Work out the finished part from the listing and answer in its coordinate system (mm). Face numbers are marked on the shaded views. A direction names the side the tool comes from. Give positions to 0.01 mm unless a question says otherwise; leave off trailing zeros. Order: outer loops, then holes, each group sorted by start corner. A loop starts at its lowest first (then second) coordinate and runs counter-clockwise, first axis right, second up. Notation, with made-up numbers: M -2,-20 L 21,-20 A17 cw 21,-3 Z; hole C 25.5,-30 d9. An arc over 180 degrees is marked long. One line per item, written item: value.
Autodesk Inventor part; units mm, degrees
ref_plane "Work Plane1" through (0, -50, 20) normal (0, -1, 0) x (0, 0, -1)
ref_plane "YZ Plane" through (0, 0, 0) normal (1, 0, 0) x (0, 1, 0)
ref_plane "XZ Plane" through (0, 0, 0) normal (0, 1, 0) x (-1, 0, 0)
sketch "Sketch1" plane through (0, 0, 0) normal (1, 0, 0) x (0, 1, 0)
  arc A0 (-15, -20) -> (-15, 20) centre (0, 0) ccw
  line L0 (-15, 20) -> (-50, 20)
  line L1 (-15, -20) -> (-50, -20)
  circle A1 centre (0, 0) radius 11.5 construction
  line L2 (25, 0) -> (0, 0) construction
  line L3 (0, 0) -> (-7.125, 12.3409) construction
  line L4 (0, 0) -> (-7.125, -12.3409) construction
  line L5 (-15, 20) -> (-15, -20) construction
  circle A2 centre (11.5, 0) radius 1.65
  circle A3 centre (-5.75, 9.9593) radius 1.65
  circle A4 centre (-5.75, -9.9593) radius 1.65
  circle A5 centre (11.5, 0) radius 2.75
  circle A6 centre (-5.75, -9.9593) radius 2.75
  circle A7 centre (-5.75, 9.9593) radius 2.75
  line L6 (0, 0) -> (5.8575, 10.1455) construction
  line L7 (0, 0) -> (5.8575, -10.1455) construction
  circle A8 centre (0, 0) radius 9.715 construction
  circle A9 centre (4.8575, 8.4134) radius 2
  circle A10 centre (4.8575, -8.4134) radius 2
  circle A11 centre (-9.715, 0) radius 2
  line L8 (-50, 20) -> (-50, -20) construction
  line L9 (-50, -20) -> (-50, 20)
  line L10 (0, 25) -> (0, -25) construction
  point P0 (-15, 0)
  dimension "d6" = 4
  dimension "d0" = 23
  dimension "d1" = 30
  dimension "d2" = 3.3
  dimension "d3" = 5.5
  dimension "d4" = 30
  dimension "d5" = 19.43
  dimension "d7" = 50
  dimension "d18" = 50
  dimension "d19" = 40
extrude "Extrusion1" add sketch "Sketch1" along normal mid plane 40 contours L1 L9 L0 A0 | A5 | A6 | A7 | A9 | A10 | A11
extrude "Extrusion2" cut sketch "Sketch1" against normal blind 35 from surface at 20 contours A5 | A6 | A7
extrude "Extrusion3" cut sketch "Sketch1" along normal blind 5 from surface at -20 contours A9 | A10 | A11
ref_plane "Work Plane1" through (0, -50, 20) normal (0, -1, 0) x (0, 0, -1)
mirror "Mirror1" about plane through (0, -50, 20) normal (0, -1, 0)
fillet "Fillet1" radius 5 12 edges at (-20, -125, 0) (-20, -50, -20) (-20, 25, 0) (-20, -50, 20) (20, -125, 0) (20, -50, -20) (20, 25, 0) (20, -50, 20) (0, -15, 20) (0, -85, 20) (0, -85, -20) (0, -15, -20)
equation "\"d18\" = 0.5 * thigh_length"
properties part number "thigh"
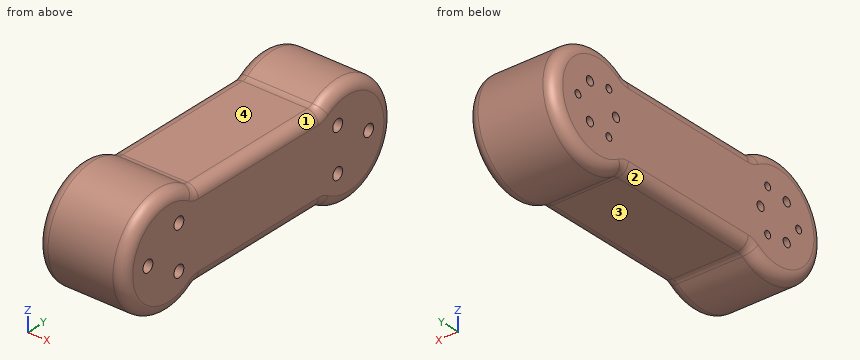
(1) Which of the six approach directions +Z, -Z, +X, -X, +Y, -Y give full straight-line access (tool end or side, diameter ignored) to the marked faces 1, 2, 3 and 4?
Findings:
face 1: +Z, +X
face 2: -Z, -X
face 3: -Z, +X, -X
face 4: +Z, +X, -X
(2) Section C-C, the plane x = 17.5 is taken. Give the vertices of the cut face in (y, z).
Findings:
outline: M -86.55,-20.28 A5.67 cw -83.42,-19.33 L -16.58,-19.33 A5.67 cw -13.45,-20.28 A24.33 ccw long -13.45,20.28 A5.67 cw -16.58,19.33 L -83.42,19.33 A5.67 cw -86.55,20.28 A24.33 ccw long Z; hole C -111.5,0 d5.5; hole C -94.25,-9.96 d5.5; hole C -94.25,9.96 d5.5; hole C -5.75,-9.96 d5.5; hole C -5.75,9.96 d5.5; hole C 11.5,0 d5.5
(3) Section A-A, the plane z = 0 is taken. Give the number of separate pieces and of enclosed holes in the cut face, then the cut area to 3 significant figures.
Findings:
separate pieces: 3
enclosed holes: 0
area: 5,520 mm^2
(4) Find the intervals of material crossed by probe 1 along Z at (x, y) = (2.5, -5.75); probe 2 along Y at (x, z) = (-6, -8.5); probe 3 along Y at (x, z) = (-3, -2), in increasing order. Write a range as from..to.
Findings:
probe 1: z = -24.33..-12.71, -7.21..7.21, 12.71..24.33
probe 2: y = -123.51..-96.58, -91.92..-8.08, -3.42..23.51
probe 3: y = -124.92..-113.39, -109.61..9.61, 13.39..24.92
(5) Given P1, Ø2, axis at y = 5.5, z = -9, coming from the -X side; P2, Ø1.6, axis at y = 11.5, z = 0, coming from the +X side; P3, Ø5, axis at x = -1.5, y = -52.5, coming from the +Z side; P4, Ø3, axis at x = -11, y = -99.5, coming from the -Z side, each flat-ended and moving along its own axis, determine where each tip first touches the part or whether it passes through.
Findings:
P1: stops at x = -15
P2: passes through
P3: stops at z = 20
P4: stops at z = -25
(6) Section B-B, the plane y = -62 is taken. Give the vertices of the cut face in (x, z).
Findings:
outline: M -20,-15 A5 ccw -15,-20 L 15,-20 A5 ccw 20,-15 L 20,15 A5 ccw 15,20 L -15,20 A5 ccw -20,15 Z
